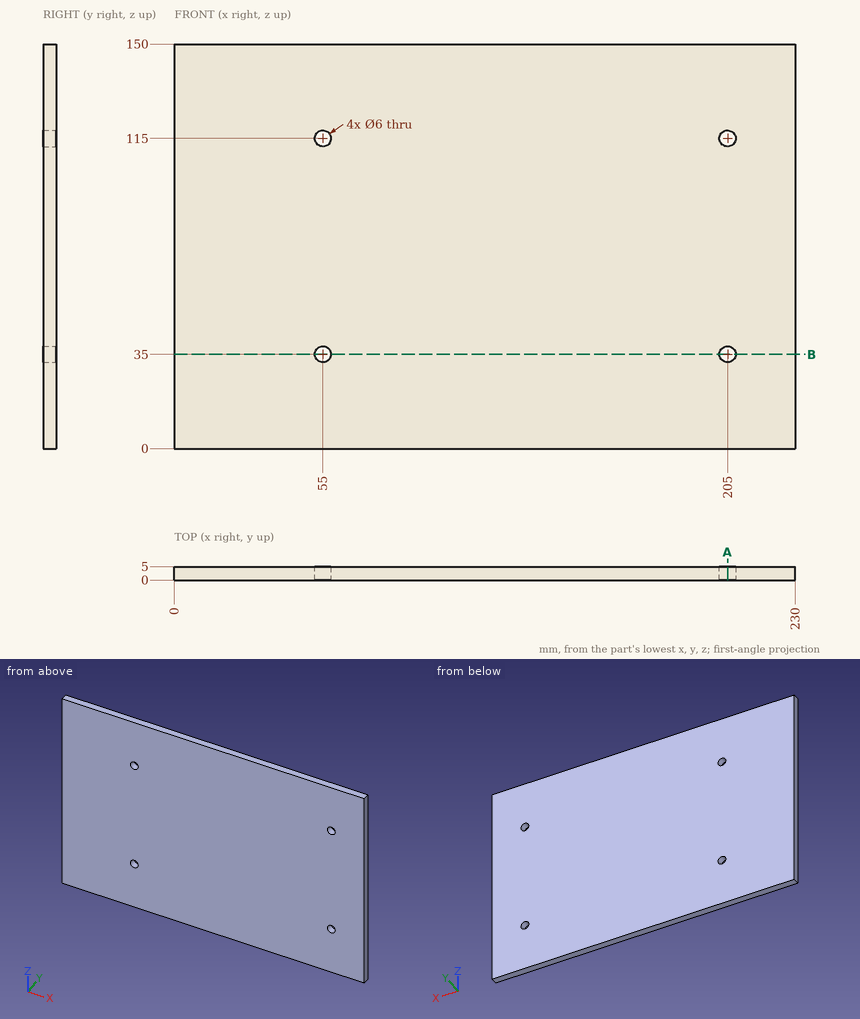
Design review of the part shown in the three views and the two pictorial views. Dimensions are in mm from the part's minimum x, y and z. Coordinates: 2 decimals unless noted, no trailing zeros. Order: outer loops, then holes, each group sorted by start corner. A loop starts at its lowest first (then second) coordinate and runs counter-clockwise, first axis right, second up.
Item 1: Take a section at B-B, the plane z = 35. Write out the cut boundary in (x, y), then the cut area to 3 significant figures.
Item 2: For line 1 (Z direction, x = 55, y = 3.95); line 2 (X direction, y = 1.3, z = 35), list the stretches that pass through material, from the lowest coordinate up.
Item 3: Take a section at A-A, the plane x = 205. Write out the cut boundary in (y, z), then the cut area to 3 significant figures.
Item 4: For pin 1 Ø5 at (x, z) = (55, 115) entering from -Y, flat-tipped, find the tip position at first contact; note if it passes through.
The answers:
1. outline: (0, 0) - (52, 0) - (52, 5) - (0, 5) - close; (58, 0) - (202, 0) - (202, 5) - (58, 5) - close; (208, 0) - (230, 0) - (230, 5) - (208, 5) - close
1. area: 1,090 mm2
2. line 1: z = 0 to 32, 38 to 112, 118 to 150
2. line 2: x = 0 to 52, 58 to 202, 208 to 230
3. outline: (0, 0) - (5, 0) - (5, 32) - (0, 32) - close; (0, 38) - (5, 38) - (5, 112) - (0, 112) - close; (0, 118) - (5, 118) - (5, 150) - (0, 150) - close
3. area: 690 mm2
4. pin 1: passes through
